```python
from build123d import *

# Parameters (mm, degrees)
SKETCH1_W               = 25.4
SKETCH1_H               = 50.8
SKETCH1_W_2             = 20.32
SKETCH1_H_2             = 45.72
EXTRUDE_THIN1_DEPTH     = 171.45
SKETCH2_R               = 2.4765
CUT_EXTRUDE1_DEPTH      = 13.7
CUT_EXTRUDE1_DEPTH_BACK = 13.7


with BuildPart() as part:
    # Sketch1 → Extrude-Thin1 (new body, symmetric)
    with BuildSketch(Plane.XY):
        Rectangle(SKETCH1_W, SKETCH1_H)
        Rectangle(SKETCH1_W_2, SKETCH1_H_2, mode=Mode.SUBTRACT)
    extrude(amount=EXTRUDE_THIN1_DEPTH, both=True)

    # Sketch2 → Cut-Extrude1 (cut, two sides)
    with BuildSketch(Plane(origin=(0, 0, 0), x_dir=(0, 0, -1), z_dir=(1, 0, 0))) as cut_extrude1_sk:
        with Locations((133.35, 12.7)):
            Circle(SKETCH2_R)
        with Locations((133.35, -12.7)):
            Circle(SKETCH2_R)
        with Locations((158.75, -12.7)):
            Circle(SKETCH2_R)
        with Locations((158.75, 12.7)):
            Circle(SKETCH2_R)
        with Locations((-133.35, 12.7)):
            Circle(SKETCH2_R)
        with Locations((-158.75, 12.7)):
            Circle(SKETCH2_R)
        with Locations((-158.75, -12.7)):
            Circle(SKETCH2_R)
        with Locations((-133.35, -12.7)):
            Circle(SKETCH2_R)
    extrude(amount=CUT_EXTRUDE1_DEPTH, mode=Mode.SUBTRACT)
    extrude(cut_extrude1_sk.sketch, amount=-CUT_EXTRUDE1_DEPTH_BACK, mode=Mode.SUBTRACT)


solid = part.part
```
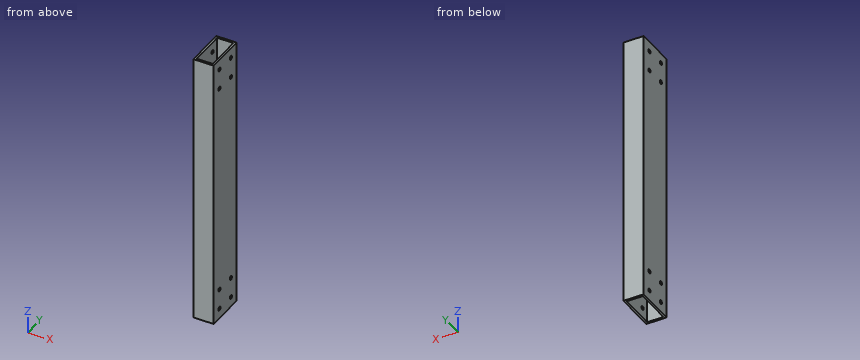
Work out the finished part from the listing and answer in its coordinate system (mm). Coordinates: 2 decimals unless noted, no trailing zeros. Loops run counter-clockwise (first coordinate to the right, second up) from the corner with the lowest first, then second, coordinate; pieces in that order, holes last.
1) Consider probe 1 along Z at (x, y) = (11.3, 12.7); probe 2 along Y at (x, z) = (11, -158.75); probe 3 along X at (y, z) = (11.5, -24). Determine where each line is inside the solid, lowest interval first.
Results:
probe 1: z = -171.45 to -161.23, -156.27 to -135.83, -130.87 to 130.87, 135.83 to 156.27, 161.23 to 171.45
probe 2: y = -25.4 to -15.18, -10.22 to 10.22, 15.18 to 25.4
probe 3: x = -12.7 to -10.16, 10.16 to 12.7
2) Flat-ended cylindrical pins translate along their axes: pin 1 (6.5 mm diameter, centred on y = -12.7, z = 158.75, fed in from -X); pin 2 (8 mm diameter, centred on x = 4, y = 5.5, fed in from +Z). Find the tip coordinate at first contact, or state that the pin passes through.
Results:
pin 1: stops at x = -12.7
pin 2: passes through
3) Section C-C (z = 148.5) is taken. Give the vertices of the cut face in (x, y).
Results:
outline: (-12.7, -25.4) - (12.7, -25.4) - (12.7, 25.4) - (-12.7, 25.4) - close; hole (-10.16, -22.86) - (10.16, -22.86) - (10.16, 22.86) - (-10.16, 22.86) - close
4) Section B-B (x = -0.25) is taken. Give the vertices of the cut face in (y, z), plus the area to 3 significant figures.
Results:
outline: (-25.4, -171.45) - (-22.86, -171.45) - (-22.86, 171.45) - (-25.4, 171.45) - close; (22.86, -171.45) - (25.4, -171.45) - (25.4, 171.45) - (22.86, 171.45) - close
area: 1,740 mm2
5) Section A-A (y = 18.5) is taken. Give the vertices of the cut face in (x, z).
Results:
outline: (-12.7, -171.45) - (-10.16, -171.45) - (-10.16, 171.45) - (-12.7, 171.45) - close; (10.16, -171.45) - (12.7, -171.45) - (12.7, 171.45) - (10.16, 171.45) - close
